from build123d import *

# Parameters (mm, degrees)
CROQUIS1_W                          = 31
CROQUIS1_H                          = 72
SALIENTE_EXTRUIR1_DEPTH             = 28
CROQUIS2_W                          = 27
CROQUIS2_H                          = 69
CORTAR_EXTRUIR1_DEPTH               = 83.170554337
CROQUIS5_W                          = 13
CROQUIS5_H                          = 10
DI_METRO_DE_TALADRO_2_5_2_5_2_D     = 2.5
DI_METRO_DE_TALADRO_2_5_2_5_2_DEPTH = 11
REDONDEO3_R                         = 5
REDONDEO4_R                         = 3
SALIENTE_EXTRUIR2_START             = 10
CROQUIS14_R                         = 13
SALIENTE_EXTRUIR2_DEPTH             = 10
CROQUIS15_W                         = 28
CROQUIS15_H                         = 82
SALIENTE_EXTRUIR3_DEPTH             = 6
CORTAR_EXTRUIR2_REACH               = 80.511
CROQUIS16_R                         = 3.55
CROQUIS17_R                         = 3.55
SALIENTE_EXTRUIR4_DEPTH             = 6
CORTAR_EXTRUIR3_DEPTH               = 88.475710915
SALIENTE_EXTRUIR5_START             = 10
SALIENTE_EXTRUIR5_DEPTH             = 10
REDONDEO5_R                         = 10
CROQUIS20_R                         = 2.25
CORTAR_EXTRUIR4_DEPTH               = 86.094065614
CROQUIS21_R                         = 4
CROQUIS21_R_2                       = 2.25
CORTAR_EXTRUIR5_DEPTH               = 3.15
SALIENTE_EXTRUIR6_START             = 2
CROQUIS22_R                         = 12.75
CROQUIS22_R_2                       = 1.25
CROQUIS22_R_3                       = 3.55
SALIENTE_EXTRUIR6_DEPTH             = 2
SALIENTE_EXTRUIR7_START             = -8
SALIENTE_EXTRUIR7_DEPTH             = 8
SALIENTE_EXTRUIR8_DEPTH             = 2
SALIENTE_EXTRUIR9_START             = 2
SALIENTE_EXTRUIR9_DEPTH             = 2
SALIENTE_EXTRUIR10_DEPTH            = 11
CROQUIS27_R                         = 12.3
CORTAR_EXTRUIR6_DEPTH               = 8
SALIENTE_EXTRUIR11_START            = 15
SALIENTE_EXTRUIR11_DEPTH            = 15
CHAFL_N1_SIZE                       = 0.5


with BuildPart() as part:
    # Croquis1 → Saliente-Extruir1 (new body)
    with BuildSketch(Plane(origin=(14, 0, 0), x_dir=(0, 0, -1), z_dir=(1, 0, 0))):
        with Locations((-12.5, 36)):
            Rectangle(CROQUIS1_W, CROQUIS1_H)
    extrude(amount=-SALIENTE_EXTRUIR1_DEPTH)

    # Croquis2 → Cortar-Extruir1 (cut, through all)
    with BuildSketch(Plane.ZY.offset(14)):
        with Locations((14.5, 35.5)):
            Rectangle(CROQUIS2_W, CROQUIS2_H)
    extrude(amount=-CORTAR_EXTRUIR1_DEPTH, mode=Mode.SUBTRACT)

    # Croquis5 → Revolución3 (revolve)
    with BuildSketch(Plane(origin=(0, 0, 14), x_dir=(-1, 0, 0), z_dir=(0, 0, -1)), mode=Mode.PRIVATE) as revoluci_n3_sk:
        with Locations((-6.5, -5)):
            Rectangle(CROQUIS5_W, CROQUIS5_H)
    revolve(revoluci_n3_sk.sketch.rotate(Axis((0, -10, 14), (0, 1, 0)), 180), axis=Axis((0, -10, 14), (0, 1, 0)))

    # Croquis6 → Cortar-Revolución1 (revolve, cut)
    with BuildSketch(Plane(origin=(0, 0, 14), x_dir=(-1, 0, 0), z_dir=(0, 0, -1)), mode=Mode.PRIVATE) as cortar_revoluci_n1_sk:
        Polygon((-12.75, -10), (0, -10), (0, 2), (-2.3, 2), (-2.3, 1), (-2.25, 1), (-2.25, 0), (-12.75, 0), align=None)
    revolve(cortar_revoluci_n1_sk.sketch.rotate(Axis((0, -10, 14), (0, 1, 0)), 180), axis=Axis((0, -10, 14), (0, 1, 0)), mode=Mode.SUBTRACT)

    # Diámetro de taladro Ø2.5 (2.5)2
    with Locations(Plane(origin=(0, 1, 0), x_dir=(1, 0, 0), z_dir=(0, 1, 0))):
        with Locations((8.5, -14), (-8.5, -14)):
            Hole(DI_METRO_DE_TALADRO_2_5_2_5_2_D / 2, depth=DI_METRO_DE_TALADRO_2_5_2_5_2_DEPTH)

    # Redondeo3
    redondeo3_edges = [part.edges().sort_by_distance(p)[0] for p in [
        (0, 1, 1),
        (0, 70, 1),
    ]]
    fillet(redondeo3_edges, radius=REDONDEO3_R)

    # Redondeo4
    redondeo4_edges = [part.edges().sort_by_distance(p)[0] for p in [
        (14, 0.5, 28),
        (-14, 0.5, 28),
        (14, 71, 28),
        (-14, 71, 28),
    ]]
    fillet(redondeo4_edges, radius=REDONDEO4_R)

    # Croquis14 → Saliente-Extruir2 (add)
    with BuildSketch(Plane.XZ.offset(SALIENTE_EXTRUIR2_START)):
        with BuildLine():
            Line((11, 28), (-11, 28))
            ThreePointArc((-11, 28), (-13.121320344, 27.121320344), (-14, 25))
            Line((-14, 25), (-14, -3))
            Line((-14, -3), (14, -3))
            Line((14, -3), (14, 25))
            ThreePointArc((14, 25), (13.121320344, 27.121320344), (11, 28))
        make_face()
        with Locations((0, 14)):
            Circle(CROQUIS14_R, mode=Mode.SUBTRACT)
    extrude(amount=-SALIENTE_EXTRUIR2_DEPTH)

    # Croquis15 → Saliente-Extruir3 (add)
    with BuildSketch(Plane(origin=(0, 0, -3), x_dir=(-1, 0, 0), z_dir=(0, 0, -1))):
        with Locations((0, 31)):
            Rectangle(CROQUIS15_W, CROQUIS15_H)
    extrude(amount=SALIENTE_EXTRUIR3_DEPTH)

    # Cortar-Extruir2: up to this face of the body (flat: up to its plane)
    cortar_extruir2_end = Plane(part.part.faces().sort_by_distance((0, 72, 9.433270582))[0])
    # Croquis16 → Cortar-Extruir2 (cut, up to the picked face)
    with BuildSketch(Plane.XZ, mode=Mode.PRIVATE) as cortar_extruir2_sk1:
        with Locations((0, 14)):
            Circle(CROQUIS16_R)
    cortar_extruir2_tool1 = split(extrude(cortar_extruir2_sk1.sketch, amount=-CORTAR_EXTRUIR2_REACH, mode=Mode.PRIVATE), bisect_by=cortar_extruir2_end, keep=Keep.BOTH, mode=Mode.PRIVATE)
    add(cortar_extruir2_tool1.solids().sort_by(Axis((0, 0, 14), (0, 1, 0)))[0], mode=Mode.SUBTRACT)

    # Croquis17 → Saliente-Extruir4 (add)
    with BuildSketch(Plane(origin=(0, 72, 0), x_dir=(1, 0, 0), z_dir=(0, 1, 0))):
        with BuildLine():
            Line((-11, -28), (11, -28))
            ThreePointArc((11, -28), (13.121320344, -27.121320344), (14, -25))
            Line((14, -25), (14, 9))
            Line((14, 9), (-14, 9))
            Line((-14, 9), (-14, -25))
            ThreePointArc((-14, -25), (-13.121320344, -27.121320344), (-11, -28))
        make_face()
        with Locations((0, -14)):
            Circle(CROQUIS17_R, mode=Mode.SUBTRACT)
    extrude(amount=SALIENTE_EXTRUIR4_DEPTH)

    # Croquis18 → Cortar-Extruir3 (cut, through all)
    with BuildSketch(Plane.ZY.offset(14)):
        with BuildLine():
            Line((6, 70), (1, 70))
            ThreePointArc((1, 70), (-1.828427125, 68.828427125), (-3, 66))
            Line((-3, 66), (-3, 5))
            ThreePointArc((-3, 5), (-1.828427125, 2.171572875), (1, 1))
            Line((1, 1), (6, 1))
            ThreePointArc((6, 1), (2.464466094, 2.464466094), (1, 6))
            Line((1, 6), (1, 65))
            ThreePointArc((1, 65), (2.464466094, 68.535533906), (6, 70))
        make_face()
    extrude(amount=-CORTAR_EXTRUIR3_DEPTH, mode=Mode.SUBTRACT)

    # Croquis19 → Saliente-Extruir5 (add)
    with BuildSketch(Plane.XZ.offset(10).offset(SALIENTE_EXTRUIR5_START)):
        with BuildLine():
            Line((-11.25, 8), (-14, 8))
            Line((-14, 8), (-14, -9))
            Line((-14, -9), (14, -9))
            Line((14, -9), (14, 8))
            Line((14, 8), (11.25, 8))
            ThreePointArc((11.25, 8), (0, 1.25), (-11.25, 8))
        make_face()
    extrude(amount=-SALIENTE_EXTRUIR5_DEPTH)

    # Redondeo5
    # the kernel refuses this fillet: 10 mm, written as the material it adds along each edge
    with BuildSketch(Plane(origin=(14, -10, 8), x_dir=(0, -1, 0), z_dir=(-1, 0, 0))) as redondeo5_piece_1_section:
        with BuildLine():
            CenterArc((REDONDEO5_R, REDONDEO5_R), REDONDEO5_R, 180, 90)
            Line((0, REDONDEO5_R), (0, 0))
            Line((0, 0), (REDONDEO5_R, 0))
        make_face()
    redondeo5_piece_1 = extrude(amount=27.75, mode=Mode.PRIVATE)
    redondeo5_piece_1 = redondeo5_piece_1 - Plane(origin=(0, -12.512239399, 14), x_dir=(-1, 0, 0), z_dir=(0, -1, 0)) * Cylinder(12.75, 96, mode=Mode.PRIVATE)
    add(redondeo5_piece_1)
    with BuildSketch(Plane(origin=(13.75, -10, 8), x_dir=(0, -1, 0), z_dir=(-1, 0, 0))) as redondeo5_piece_2_section:
        with BuildLine():
            CenterArc((REDONDEO5_R, REDONDEO5_R), REDONDEO5_R, 180, 90)
            Line((0, REDONDEO5_R), (0, 0))
            Line((0, 0), (REDONDEO5_R, 0))
        make_face()
    redondeo5_piece_2 = extrude(amount=27.75, mode=Mode.PRIVATE)
    redondeo5_piece_2 = redondeo5_piece_2 - Plane(origin=(0, -12.552647231, 14), x_dir=(-1, 0, 0), z_dir=(0, -1, 0)) * Cylinder(12.75, 96, mode=Mode.PRIVATE)
    add(redondeo5_piece_2)

    # Croquis20 → Cortar-Extruir4 (cut, through all)
    with BuildSketch(Plane.XY.offset(-3)):
        with Locations((0, 51)):
            Circle(CROQUIS20_R)
        with Locations((0, 20)):
            Circle(CROQUIS20_R)
    extrude(amount=-CORTAR_EXTRUIR4_DEPTH, mode=Mode.SUBTRACT)

    # Croquis21 → Cortar-Extruir5 (cut)
    # profile 1 of 2: a face of its own
    with BuildSketch(Plane.XY.offset(-3)):
        with Locations((0, 51)):
            Circle(CROQUIS21_R)
        with Locations((0, 51)):
            Circle(CROQUIS21_R_2, mode=Mode.SUBTRACT)
    # profile 2 of 2: a face of its own
    with BuildSketch(Plane.XY.offset(-3)):
        with Locations((0, 20)):
            Circle(CROQUIS21_R)
        with Locations((0, 20)):
            Circle(CROQUIS21_R_2, mode=Mode.SUBTRACT)
    extrude(amount=-CORTAR_EXTRUIR5_DEPTH, mode=Mode.SUBTRACT)

    # Croquis22 → Saliente-Extruir6 (add)
    with BuildSketch(Plane.XZ.offset(SALIENTE_EXTRUIR6_START)):
        with Locations(Location((0, 14, 0), (0, 0, 161.71611006))):
            Circle(CROQUIS22_R)
        with Locations(Location((8.5, 14, 0), (0, 0, 90))):
            Circle(CROQUIS22_R_2, mode=Mode.SUBTRACT)
        with Locations((0, 14)):
            Circle(CROQUIS22_R_3, mode=Mode.SUBTRACT)
        with Locations(Location((-8.5, 14, 0), (0, 0, 90))):
            Circle(CROQUIS22_R_2, mode=Mode.SUBTRACT)
    extrude(amount=-SALIENTE_EXTRUIR6_DEPTH)

    # Croquis23 → Saliente-Extruir7 (add)
    with BuildSketch(Plane(origin=(0, 78, 0), x_dir=(1, 0, 0), z_dir=(0, 1, 0)).offset(SALIENTE_EXTRUIR7_START)):
        with BuildLine():
            Line((-11, -30), (11, -30))
            ThreePointArc((11, -30), (14.535533906, -28.535533906), (16, -25))
            Line((16, -25), (16, 9))
            Line((16, 9), (14, 9))
            Line((14, 9), (14, -25))
            ThreePointArc((14, -25), (13.121320344, -27.121320344), (11, -28))
            Line((11, -28), (-11, -28))
            ThreePointArc((-11, -28), (-13.121320344, -27.121320344), (-14, -25))
            Line((-14, -25), (-14, 9))
            Line((-14, 9), (-16, 9))
            Line((-16, 9), (-16, -25))
            ThreePointArc((-16, -25), (-14.535533906, -28.535533906), (-11, -30))
        make_face()
    extrude(amount=SALIENTE_EXTRUIR7_DEPTH)

    # Croquis24 → Saliente-Extruir8 (add)
    with BuildSketch(Plane.ZY.offset(14)):
        with BuildLine():
            Line((1, 70), (-9, 70))
            Line((-9, 70), (-9, -20))
            Line((-9, -20), (8, -20))
            ThreePointArc((8, -20), (10.928932188, -12.928932188), (18, -10))
            Line((18, -10), (25, -10))
            Line((25, -10), (25, 1))
            Line((25, 1), (1, 1))
            ThreePointArc((1, 1), (-1.828427125, 2.171572875), (-3, 5))
            Line((-3, 5), (-3, 66))
            ThreePointArc((-3, 66), (-1.828427125, 68.828427125), (1, 70))
        make_face()
    extrude(amount=SALIENTE_EXTRUIR8_DEPTH)

    # Croquis25 → Saliente-Extruir9 (add)
    with BuildSketch(Plane(origin=(14, 0, 0), x_dir=(0, 0, -1), z_dir=(1, 0, 0)).offset(SALIENTE_EXTRUIR9_START)):
        with BuildLine():
            Line((9, -20), (9, 70))
            Line((9, 70), (-1, 70))
            ThreePointArc((-1, 70), (1.828427125, 68.828427125), (3, 66))
            Line((3, 66), (3, 5))
            ThreePointArc((3, 5), (1.828427125, 2.171572875), (-1, 1))
            Line((-1, 1), (-25, 1))
            Line((-25, 1), (-25, -10))
            Line((-25, -10), (-18, -10))
            ThreePointArc((-18, -10), (-10.928932188, -12.928932188), (-8, -20))
            Line((-8, -20), (9, -20))
        make_face()
    extrude(amount=-SALIENTE_EXTRUIR9_DEPTH)

    # Croquis26 → Saliente-Extruir10 (add)
    with BuildSketch(Plane.XZ.offset(10)):
        with BuildLine():
            Line((11, 30), (-11, 30))
            ThreePointArc((-11, 30), (-14.535533906, 28.535533906), (-16, 25))
            Line((-16, 25), (-14, 25))
            ThreePointArc((-14, 25), (-13.121320344, 27.121320344), (-11, 28))
            Line((-11, 28), (11, 28))
            ThreePointArc((11, 28), (13.121320344, 27.121320344), (14, 25))
            Line((14, 25), (16, 25))
            ThreePointArc((16, 25), (14.535533906, 28.535533906), (11, 30))
        make_face()
    extrude(amount=-SALIENTE_EXTRUIR10_DEPTH)

    # Croquis27 → Cortar-Extruir6 (cut)
    with BuildSketch(Plane(origin=(0, 78, 0), x_dir=(1, 0, 0), z_dir=(0, 1, 0))):
        with Locations(Location((0, -14, 0), (0, 0, 270))):
            Circle(CROQUIS27_R)
    extrude(amount=-CORTAR_EXTRUIR6_DEPTH, mode=Mode.SUBTRACT)

    # Croquis28 → Saliente-Extruir11 (add)
    with BuildSketch(Plane.XZ.offset(20).offset(SALIENTE_EXTRUIR11_START)):
        with BuildLine():
            Line((16, 8), (11.25, 8))
            ThreePointArc((11.25, 8), (0, 1.25), (-11.25, 8))
            Line((-11.25, 8), (-16, 8))
            Line((-16, 8), (-16, -9))
            Line((-16, -9), (16, -9))
            Line((16, -9), (16, 8))
        make_face()
    extrude(amount=-SALIENTE_EXTRUIR11_DEPTH)

    # Chaflán1
    chafl_n1_edges = [part.edges().sort_by_distance(p)[0] for p in [
        (0, 78, 1.7),
    ]]
    chamfer(chafl_n1_edges, length=CHAFL_N1_SIZE)


solid = part.part
The model under review builds one solid part; all positions refer to its coordinate system, in mm. A direction names the side the tool comes from. Round coordinates to 2 decimals unless told otherwise and drop trailing zeros. Loops run counter-clockwise (first coordinate to the right, second up) from the corner with the lowest first, then second, coordinate; pieces in that order, holes last. Notation, with made-up numbers: M 1,75 L 28,75 A19 cw 28,92 Z; hole C -18,49 d1. An arc over 180 degrees is marked long. Answer as CSV lines item,"result". Start each with the question number.
Item 1: Consider section D-D (y = -26). Write out the cut boundary in (x, z).
Item 2: For faces 5 (the face through (0, -10, 27)), 6 (the face through (0.224, 68.859, -1.797)), 7 (the face through (-1.7, -2, 17.4)), 8 (the face through (-7.484, 73.802, 4.239)), list the 3-axis set-ups (+Z, -Z, +X, -X, +Y, -Y) from which the entire face can be reached by the end or side of a thin tool; tool diameter is ignored.
Item 3: Consider section C-C (z = 14). State how many separate pieces and enclosed holes the cut face has, then the cut area to 3 significant figures.
Item 4: Wall thickness on line 1 (Y direction, x = 0, z = -7.45); line 2 (Z direction, x = -8.5, y = -0.8); line 3 (Y direction, x = 10, z = 5.5): over which ranges is each line inside the solid? List them lowest first. Write a range as [from, to].
Item 5: Consider section A-A (y = 51). Write out the cut boundary in (x, z).
Item 6: Consider section B-B (y = -7.5). Write out the cut boundary in (x, z), then the cut area to 3 significant figures.
Item 7: Insertion check: P1, Ø2.5, axis at x = -14.5, y = -27.5, coming from the +Z side; P2, Ø4, axis at x = 2, y = 50, coming from the +Z side; P3, Ø2.5, axis at x = -1.5, y = 18.5, coming from the +Z side. Each pin has a flat end and moves straight along its axis. Give the tip position at first contact, or say it passes through.
Item 8: Mouldability with a two-part tool opening along X and no side actions: class faces 1 (the face through (15, -5, 28)), 2 (the face through (-16, 21, -7)), 3 (the face through (-0.244, -15.064, 1.252)), 4 (the face through (0, -35, -2)) as released by +X, released by -X, zero draft, split by the parting line, or undercut.
Answer:
1,outline,"M -16,-9 L 16,-9 L 16,8 L 11.25,8 A12.75 cw -11.25,8 L -16,8 Z"
2,face 5,"+Z, +X, -X, -Y"
2,face 6,"+Z, +X, -X"
2,face 7,"-Y"
2,face 8,"+Y"
3,separate pieces,"6"
3,enclosed holes,"0"
3,area,"176 mm^2"
4,line 1,"y = [-35, 17.75], [22.25, 48.75], [53.25, 78]"
4,line 2,"z = [-9, 12.75], [15.25, 30]"
4,line 3,"y = [-35, 1], [70, 78]"
5,outline,"M -16,-9 L -2.25,-9 L -2.25,-6.15 L -4,-6.15 L -4,-3 L -16,-3 Z; M 2.25,-9 L 16,-9 L 16,-3 L 4,-3 L 4,-6.15 L 2.25,-6.15 Z"
6,outline,"M -16,-9 L 16,-9 L 16,25 A5 ccw 11,30 L -11,30 A5 ccw -16,25 Z; hole C 0,14 d25.5"
6,area,"727 mm^2"
7,P1,"stops at z = 8"
7,P2,"stops at z = -3"
7,P3,"stops at z = -6.15"
8,face 1,"released by +X"
8,face 2,"released by -X"
8,face 3,"undercut"
8,face 4,"zero draft"
